Geometry check sheet. Reference: the model listing, model coordinates, mm. Face numbers are marked on the shaded views. A direction names the side the tool comes from. Give positions to 0.01 mm unless a question says otherwise; leave off trailing zeros. Order: outer loops, then holes, each group sorted by start corner. A loop starts at its lowest first (then second) coordinate and runs counter-clockwise, first axis right, second up. Notation, with made-up numbers: M 72.5,-15.5 L 125.5,-15.5 A21 ccw 125.5,14.5 Z; hole C 61.5,83 d10. An arc over 180 degrees is marked long. Answer as CSV lines item,"result". Start each with the question number.
Q1. Go/stop test with flat-tipped pins: pin 1 (12 mm diameter, centred on x = -25.5, z = -39.5, fed in from +Y); pin 2 (1 mm diameter, centred on x = 6, z = -36.5, fed in from -Y); pin 3 (2 mm diameter, centred on y = -7, z = -45.5, fed in from -X). Record where each tip stops, or that it passes through.
Q2. Section check C-C, the plane x = 0. Record the boundary of the cut face in (y, z), then the cut area to 3 significant figures.
Q3. Mould release check, pull along Y, two halves, no side actions. Record for the marked faces 1, 2, 3 and 4: +Y half, -Y half, draft (parallel to the pull), parting line (faces both ways), or undercut.
Q4. Section check D-D, the plane y = -20. Record the boundary of the cut face in (x, z).
Q5. Section check B-B, the plane x = 15. Record the boundary of the cut face in (y, z), then the cut area to 3 significant figures.
Q6. Thickness scan on line 1 (X direction, y = 0, z = -12); line 2 (X direction, y = 1, z = -36.5); line 3 (Y direction, x = 0.5, z = -48.5). Record the ranges inside material, lowest first.
Q7. Set-up check for the marked faces 5, 6 and 7: record each of +Z, -Z, +X, -X, +Y, -Y from which the full face is reachable in a straight line by a thin tool's end or side.
Q8. Section check A-A, the plane z = -50. Count the separate pieces of the cut face and the enclosed holes in it, then the cut area to 3 significant figures.
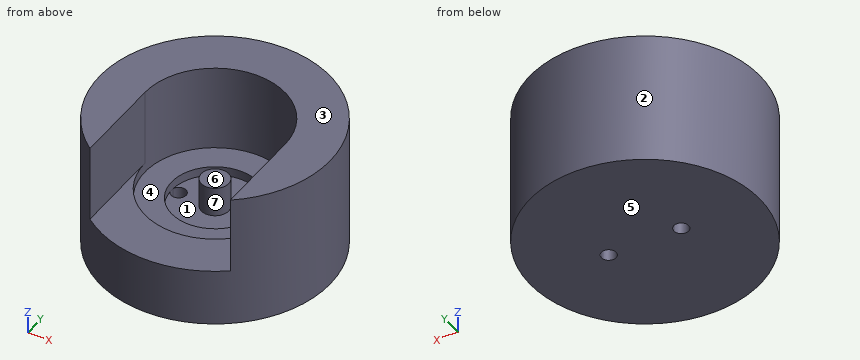
```python
from build123d import *

# Parameters (mm, degrees)
F0_R     = 49.2125
F1_DEPTH = 57.15
F2_R     = 18.542
F3_DEPTH = 40.64
F4_DEPTH = 36.83
F5_DEPTH = 32.766
F6_R     = 5.842
F7_DEPTH = 12.7
F9_DEPTH = 16.511


with BuildPart() as f1:
    # F0 (on Top) → F1 (new body)
    with BuildSketch(Plane.XY):
        Circle(F0_R)
    extrude(amount=-F1_DEPTH)

    # F2 (on face) → F3 (cut)
    with BuildSketch(Plane.XY):
        Circle(F2_R)
    extrude(amount=-F3_DEPTH, mode=Mode.SUBTRACT)

    # F2 (on face) → F4 (cut)
    with BuildSketch(Plane.XY):
        with BuildLine():
            ThreePointArc((-29.972, 0), (0, -29.972), (29.972, 0))
            ThreePointArc((29.972, 0), (0, 29.972), (-29.972, 0))
        make_face()
        Circle(F2_R, mode=Mode.SUBTRACT)
    extrude(amount=-F4_DEPTH, mode=Mode.SUBTRACT)

    # F2 (on face) → F5 (cut)
    with BuildSketch(Plane.XY):
        with BuildLine():
            Line((29.972, -39.0326705754), (29.972, 0))
            ThreePointArc((29.972, 0), (0, -29.972), (-29.972, 0))
            Line((-29.972, 0), (-29.972, -39.0326705754))
            ThreePointArc((-29.972, -39.0326705754), (0, -49.2125), (29.972, -39.0326705754))
        make_face()
    extrude(amount=-F5_DEPTH, mode=Mode.SUBTRACT)

    # F6 (on face) → F7 (join)
    with BuildSketch(Plane.XY.offset(-40.64)):
        Circle(F6_R)
    extrude(amount=F7_DEPTH)

    # F8 (on face) → F9 (cut, through all)
    with BuildSketch(Plane.XY.offset(-40.64)):
        with BuildLine():
            ThreePointArc((-18.5140256757, -1.0181440372), (-14.9907707511, -3.1328009848), (-12.3317, 0))
            ThreePointArc((-12.3317, 0), (-14.9907707511, 3.1328009848), (-18.5140256757, 1.0181440372))
            ThreePointArc((-18.5140256757, 1.0181440372), (-18.542, 0), (-18.5140256757, -1.0181440372))
        make_face()
        with BuildLine():
            ThreePointArc((18.542, 0), (18.5350050995, 0.5092641366), (18.5140256757, 1.0181440372))
            ThreePointArc((18.5140256757, 1.0181440372), (12.3317, 0), (18.5140256757, -1.0181440372))
            ThreePointArc((18.5140256757, -1.0181440372), (18.5350050995, -0.5092641366), (18.542, 0))
        make_face()
    extrude(amount=-F9_DEPTH, mode=Mode.SUBTRACT)


solid = f1.part
```
Answer block:
1,pin 1,"stops at y = 45.18"
1,pin 2,"stops at y = -48.9"
1,pin 3,"stops at x = -48.85"
2,outline,"M -49.21,-57.15 L 49.21,-57.15 L 49.21,0 L 29.97,0 L 29.97,-36.83 L 18.54,-36.83 L 18.54,-40.64 L 5.84,-40.64 L 5.84,-27.94 L -5.84,-27.94 L -5.84,-40.64 L -18.54,-40.64 L -18.54,-36.83 L -29.97,-36.83 L -29.97,-32.77 L -49.21,-32.77 Z"
2,area,"2,790 mm2"
3,face 1,"undercut"
3,face 2,"parting line"
3,face 3,"draft"
3,face 4,"undercut"
4,outline,"M -44.97,-57.15 L 44.97,-57.15 L 44.97,0 L 29.97,0 L 29.97,-32.77 L 22.32,-32.77 L 22.32,-36.83 L -22.32,-36.83 L -22.32,-32.77 L -29.97,-32.77 L -29.97,0 L -44.97,0 Z"
5,outline,"M -46.87,-57.15 L -3.13,-57.15 L -3.13,-40.64 L -10.9,-40.64 L -10.9,-36.83 L -25.95,-36.83 L -25.95,-32.77 L -46.87,-32.77 Z; M 3.13,-57.15 L 46.87,-57.15 L 46.87,0 L 25.95,0 L 25.95,-36.83 L 10.9,-36.83 L 10.9,-40.64 L 3.13,-40.64 Z"
5,area,"2,570 mm2"
6,line 1,"x = -49.21 to -29.97, 29.97 to 49.21"
6,line 2,"x = -49.2 to -29.96, -5.76 to 5.76, 29.96 to 49.2"
6,line 3,"y = -49.21 to 49.21"
7,face 5,"-Z, +X, -X, +Y, -Y"
7,face 6,"+Z, -Y"
7,face 7,"+Z"
8,separate pieces,"1"
8,enclosed holes,"2"
8,area,"7,550 mm2"
